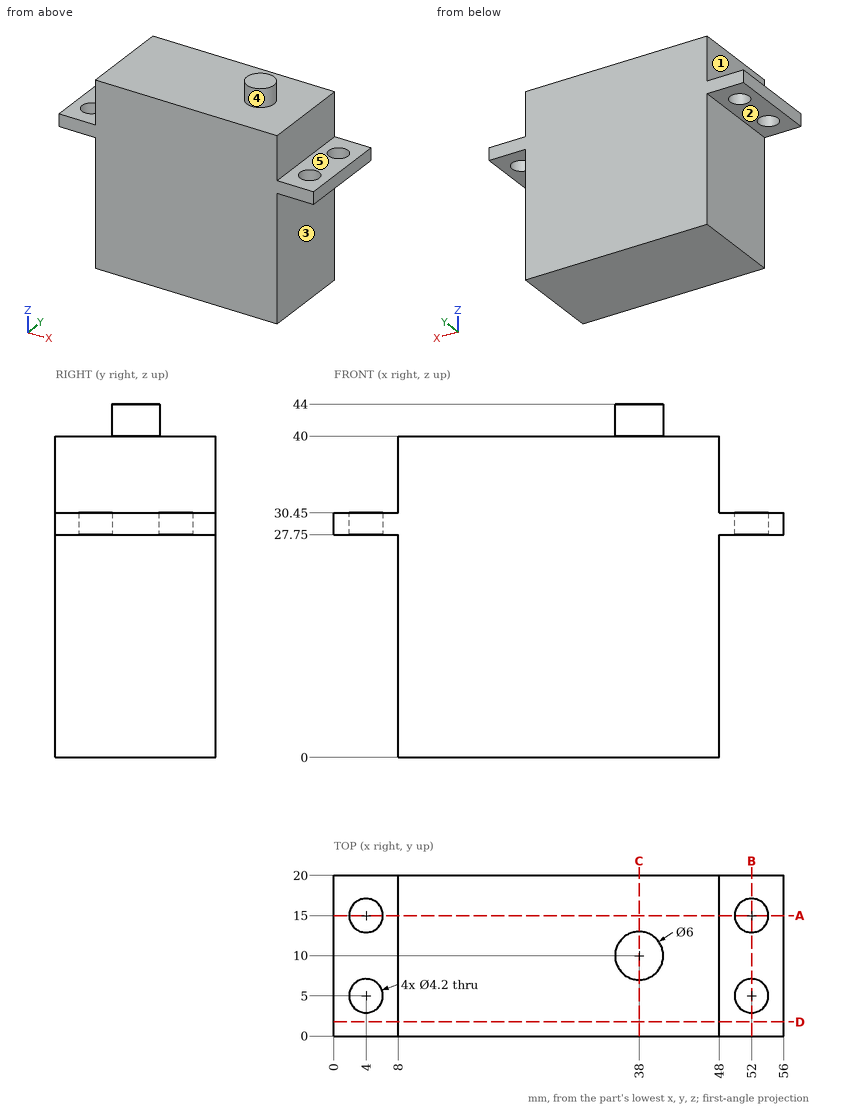
Geometry: see drawing. Coordinates: mm, zero at the bounding-box minimum. A direction names the side the tool comes from. Coordinates: 2 decimals unless noted, no trailing zeros. Loops run counter-clockwise (first coordinate to the right, second up) from the corner with the lowest first, then second, coordinate; pieces in that order, holes last.
(1) Section D-D on y = 1.75. Return the cut outline in (x, z), then the cut area to 3 significant figures.
(2) Section C-C on x = 38. Return the cut outline in (y, z).
(3) Section B-B on x = 52. Return the cut outline in (y, z).
(4) First-contact query: pin 1 Ø2.5 at (x, y) = (4, 15) entering from +Z; pin 2 Ø9 at (x, y) = (3, 10) entering from -Z; pin 3 Ø3 at (x, y) = (31.5, 5.5) entering from -Z; pin 4 Ø3 at (y, z) = (6.5, 36.5) entering from +X. Flat tips, straight axial feed; report the tip coordinate or a pass-through.
(5) Section A-A on y = 15. Return the cut outline in (x, z).
(6) Material intervals for probe 1 along Y at (x, z) = (52, 29.25); probe 2 along X at (y, z) = (15, 29.6); probe 3 along X at (y, z) = (18.5, 20.5), sorted ascending.
(7) Set-up query: the marked faces 1, 2, 3, 4 and 5. Return all of +Z, -Z, +X, -X, +Y, -Y with unobstructed straight access to the full face (end or side cutting, diameter ignored); none if empty.
Data:
1. outline: (0, 27.75) - (8, 27.75) - (8, 0) - (48, 0) - (48, 27.75) - (56, 27.75) - (56, 30.45) - (48, 30.45) - (48, 40) - (8, 40) - (8, 30.45) - (0, 30.45) - close
1. area: 1,640 mm2
2. outline: (0, 0) - (20, 0) - (20, 40) - (13, 40) - (13, 44) - (7, 44) - (7, 40) - (0, 40) - close
3. outline: (0, 27.75) - (2.9, 27.75) - (2.9, 30.45) - (0, 30.45) - close; (7.1, 27.75) - (12.9, 27.75) - (12.9, 30.45) - (7.1, 30.45) - close; (17.1, 27.75) - (20, 27.75) - (20, 30.45) - (17.1, 30.45) - close
4. pin 1: passes through
4. pin 2: stops at z = 27.75
4. pin 3: stops at z = 0
4. pin 4: stops at x = 48
5. outline: (0, 27.75) - (1.9, 27.75) - (1.9, 30.45) - (0, 30.45) - close; (6.1, 27.75) - (8, 27.75) - (8, 0) - (48, 0) - (48, 27.75) - (49.9, 27.75) - (49.9, 30.45) - (48, 30.45) - (48, 40) - (8, 40) - (8, 30.45) - (6.1, 30.45) - close; (54.1, 27.75) - (56, 27.75) - (56, 30.45) - (54.1, 30.45) - close
6. probe 1: y = 0 to 2.9, 7.1 to 12.9, 17.1 to 20
6. probe 2: x = 0 to 1.9, 6.1 to 49.9, 54.1 to 56
6. probe 3: x = 8 to 48
7. face 1: +Z, -X, +Y, -Y
7. face 2: -Z, -X, +Y, -Y
7. face 3: -Z, +X, +Y, -Y
7. face 4: +Z
7. face 5: +Z, +X, +Y, -Y
